```python
from build123d import *

# Parameters (mm, degrees)
SKETCH_1_R               = 19.5
SKETCH_1_R_2             = 18
EXTRUDE_1_DEPTH          = 20
SKETCH_3_R               = 27.5
EXTRUDE_2_DEPTH          = 3
SKETCH_10_R              = 6
SKETCH_10_R_2            = 5
EXTRUDE_6_DEPTH          = 10
CUT_EXTRUDE_4_DEPTH      = 19
CUT_EXTRUDE_4_DEPTH_BACK = 10
SKETCH_11_R              = 5.007506695
EXTRUDE_START            = 2
SKETCH_25_R              = 21.75
SKETCH_25_R_2            = 19.5
EXTRUDE_12_DEPTH         = 2
EXTRUDE_START_2          = -1
SKETCH_26_R              = 21.75
SKETCH_26_R_2            = 19.5
EXTRUDE_13_DEPTH         = 2
EXTRUDE_START_3          = -3
SKETCH_27_R              = 5.007506695
EXTRUDE_14_DEPTH         = 3
SKETCH_28_W              = 22.795630141
SKETCH_28_H              = 3
SKETCH_28_W_2            = 2.204369859
EXTRUDE_17_DEPTH         = 2
EXTRUDE_START_4          = -53
EXTRUDE_19_DEPTH         = 53
SKETCH_32_W              = 2.204369859
SKETCH_32_H              = 3
EXTRUDE_20_DEPTH         = 2
CUT_EXTRUDE_START        = -50
CUT_EXTRUDE_8_DEPTH      = 50


with BuildPart() as part:
    # Sketch 1 → Extrude 1 (new body)
    with BuildSketch(Plane(origin=(0, 0, 0), x_dir=(1, 0, 0), z_dir=(0, 1, 0))):
        with Locations(Location((0, 0, 0), (0, 0, 270))):
            Circle(SKETCH_1_R)
        with Locations(Location((0, 0, 0), (0, 0, 270))):
            Circle(SKETCH_1_R_2, mode=Mode.SUBTRACT)
    extrude(amount=EXTRUDE_1_DEPTH)

    # Sketch 3 → Extrude 2 (add)
    with BuildSketch(Plane.XZ):
        with Locations(Location((0, 0, 0), (0, 0, 270))):
            Circle(SKETCH_3_R)
    extrude(amount=EXTRUDE_2_DEPTH)

    # Sketch 10 → Extrude 6 (add)
    with BuildSketch(Plane(origin=(0, -3, 0), x_dir=(-1, 0, 0), z_dir=(0, -1, 0))):
        with Locations(Location((0, 11.196036894, 0), (0, 0, 90))):
            Circle(SKETCH_10_R)
        with Locations(Location((0, 11.196036894, 0), (0, 0, 90))):
            Circle(SKETCH_10_R_2, mode=Mode.SUBTRACT)
    extrude(amount=-EXTRUDE_6_DEPTH)

    # Sketch 11 → Cut-Extrude 4 (cut, two sides: drawn at the far end of the back side and taken through both)
    with BuildSketch(Plane(origin=(0, -3, 0), x_dir=(-1, 0, 0), z_dir=(0, -1, 0)).offset(-CUT_EXTRUDE_4_DEPTH_BACK)):
        with Locations(Location((0, 11.196036894, 0), (0, 0, 90))):
            Circle(SKETCH_11_R)
    extrude(amount=CUT_EXTRUDE_4_DEPTH + CUT_EXTRUDE_4_DEPTH_BACK, mode=Mode.SUBTRACT)

    # Sketch 25 → Extrude 12 (add)
    with BuildSketch(Plane(origin=(0, 7, 0), x_dir=(-1, 0, 0), z_dir=(0, -1, 0)).offset(EXTRUDE_START)):
        with Locations(Location((0, 0, 0), (0, 0, 90))):
            Circle(SKETCH_25_R)
        with Locations(Location((0, 0, 0), (0, 0, 90))):
            Circle(SKETCH_25_R_2, mode=Mode.SUBTRACT)
    extrude(amount=-EXTRUDE_12_DEPTH)

    # Sketch 26 → Extrude 13 (add)
    with BuildSketch(Plane(origin=(0, 10.5, 0), x_dir=(-1, 0, 0), z_dir=(0, -1, 0)).offset(EXTRUDE_START_2)):
        with Locations(Location((0, 0, 0), (0, 0, 90))):
            Circle(SKETCH_26_R)
        with Locations(Location((0, 0, 0), (0, 0, 90))):
            Circle(SKETCH_26_R_2, mode=Mode.SUBTRACT)
    extrude(amount=-EXTRUDE_13_DEPTH)

    # Sketch 27 → Extrude 14 (add)
    # profile 1 of 6: a face of its own
    with BuildSketch(Plane.XZ.offset(3).offset(EXTRUDE_START_3)):
        with BuildLine():
            Line((12.5, 0), (0, 0))
            Line((0, 0), (-12.5, 0))
            Line((-12.5, 0), (-12.5, -24.494897428))
            ThreePointArc((-12.5, -24.494897428), (-11.408888911, -25.021735628), (-10.295630141, -25.5))
            Line((-10.295630141, -25.5), (10.295630141, -25.5))
            ThreePointArc((10.295630141, -25.5), (11.408888911, -25.021735628), (12.5, -24.494897428))
            Line((12.5, -24.494897428), (12.5, 0))
        make_face()
        with Locations(Location((0, -11.196036894, 0), (0, 0, 270))):
            Circle(SKETCH_27_R, mode=Mode.SUBTRACT)
    # profile 2 of 6: a face of its own
    with BuildSketch(Plane.XZ.offset(3).offset(EXTRUDE_START_3)):
        with BuildLine():
            Line((-12.5, 0), (0, 0))
            Line((0, 0), (12.5, 0))
            Line((12.5, 0), (12.5, 24.494897428))
            ThreePointArc((12.5, 24.494897428), (11.408888911, 25.021735628), (10.295630141, 25.5))
            Line((10.295630141, 25.5), (-10.295630141, 25.5))
            ThreePointArc((-10.295630141, 25.5), (-11.408888911, 25.021735628), (-12.5, 24.494897428))
            Line((-12.5, 24.494897428), (-12.5, 0))
        make_face()
    # profile 3 of 6: a face of its own
    with BuildSketch(Plane.XZ.offset(3).offset(EXTRUDE_START_3)):
        with BuildLine():
            ThreePointArc((-10.295630141, -25.5), (-11.408888911, -25.021735628), (-12.5, -24.494897428))
            Line((-12.5, -24.494897428), (-12.5, -25.5))
            Line((-12.5, -25.5), (-10.295630141, -25.5))
        make_face()
    # profile 4 of 6: a face of its own
    with BuildSketch(Plane.XZ.offset(3).offset(EXTRUDE_START_3)):
        with BuildLine():
            Line((12.5, -25.5), (12.5, -24.494897428))
            ThreePointArc((12.5, -24.494897428), (11.408888911, -25.021735628), (10.295630141, -25.5))
            Line((10.295630141, -25.5), (12.5, -25.5))
        make_face()
    # profile 5 of 6: a face of its own
    with BuildSketch(Plane.XZ.offset(3).offset(EXTRUDE_START_3)):
        with BuildLine():
            ThreePointArc((10.295630141, 25.5), (11.408888911, 25.021735628), (12.5, 24.494897428))
            Line((12.5, 24.494897428), (12.5, 25.5))
            Line((12.5, 25.5), (10.295630141, 25.5))
        make_face()
    # profile 6 of 6: a face of its own
    with BuildSketch(Plane.XZ.offset(3).offset(EXTRUDE_START_3)):
        with BuildLine():
            Line((-12.5, 25.5), (-12.5, 24.494897428))
            ThreePointArc((-12.5, 24.494897428), (-11.408888911, 25.021735628), (-10.295630141, 25.5))
            Line((-10.295630141, 25.5), (-12.5, 25.5))
        make_face()
    extrude(amount=EXTRUDE_14_DEPTH)

    # Sketch 28 → Extrude 17 (add)
    with BuildSketch(Plane(origin=(0, 0, -25.5), x_dir=(-1, 0, 0), z_dir=(0, 0, -1))):
        with BuildLine():
            Line((12.5, -38), (12.5, -3))
            Line((12.5, -3), (10.295630141, -3))
            Line((10.295630141, -3), (-12.5, -3))
            Line((-12.5, -3), (-12.5, -38))
            Line((-12.5, -38), (-8.6, -38))
            Line((-8.6, -38), (-8.6, -37.5))
            ThreePointArc((-8.6, -37.5), (-7.1, -36), (-5.6, -37.5))
            Line((-5.6, -37.5), (-5.6, -38))
            Line((-5.6, -38), (-4, -38))
            ThreePointArc((-4, -38), (0, -34), (4, -38))
            Line((4, -38), (5.6, -38))
            Line((5.6, -38), (5.6, -37.5))
            ThreePointArc((5.6, -37.5), (7.1, -36), (8.6, -37.5))
            Line((8.6, -37.5), (8.6, -38))
            Line((8.6, -38), (12.5, -38))
        make_face()
        with Locations((-1.102184929, -1.5)):
            Rectangle(SKETCH_28_W, SKETCH_28_H)
        with Locations((11.397815071, -1.5)):
            Rectangle(SKETCH_28_W_2, SKETCH_28_H)
        with BuildLine():
            ThreePointArc((-12.5, -38), (0, -50.5), (12.5, -38))
            Line((12.5, -38), (8.6, -38))
            Line((8.6, -38), (8.6, -38.5))
            ThreePointArc((8.6, -38.5), (7.1, -40), (5.6, -38.5))
            Line((5.6, -38.5), (5.6, -38))
            Line((5.6, -38), (4, -38))
            ThreePointArc((4, -38), (0, -42), (-4, -38))
            Line((-4, -38), (-5.6, -38))
            Line((-5.6, -38), (-5.6, -38.5))
            ThreePointArc((-5.6, -38.5), (-7.1, -40), (-8.6, -38.5))
            Line((-8.6, -38.5), (-8.6, -38))
            Line((-8.6, -38), (-12.5, -38))
        make_face()
    extrude(amount=EXTRUDE_17_DEPTH)

    # Sketch 28_15 → Extrude 19 (add)
    with BuildSketch(Plane(origin=(0, 0, -25.5), x_dir=(-1, 0, 0), z_dir=(0, 0, -1)).offset(EXTRUDE_START_4)):
        with BuildLine():
            Line((12.5, -38), (12.5, -3))
            Line((12.5, -3), (10.295630141, -3))
            Line((10.295630141, -3), (-12.5, -3))
            Line((-12.5, -3), (-12.5, -38))
            Line((-12.5, -38), (-8.6, -38))
            Line((-8.6, -38), (-8.6, -37.5))
            ThreePointArc((-8.6, -37.5), (-7.1, -36), (-5.6, -37.5))
            Line((-5.6, -37.5), (-5.6, -38))
            Line((-5.6, -38), (-4, -38))
            ThreePointArc((-4, -38), (0, -34), (4, -38))
            Line((4, -38), (5.6, -38))
            Line((5.6, -38), (5.6, -37.5))
            ThreePointArc((5.6, -37.5), (7.1, -36), (8.6, -37.5))
            Line((8.6, -37.5), (8.6, -38))
            Line((8.6, -38), (12.5, -38))
        make_face()
        with BuildLine():
            ThreePointArc((-12.5, -38), (0, -50.5), (12.5, -38))
            Line((12.5, -38), (8.6, -38))
            Line((8.6, -38), (8.6, -38.5))
            ThreePointArc((8.6, -38.5), (7.1, -40), (5.6, -38.5))
            Line((5.6, -38.5), (5.6, -38))
            Line((5.6, -38), (4, -38))
            ThreePointArc((4, -38), (0, -42), (-4, -38))
            Line((-4, -38), (-5.6, -38))
            Line((-5.6, -38), (-5.6, -38.5))
            ThreePointArc((-5.6, -38.5), (-7.1, -40), (-8.6, -38.5))
            Line((-8.6, -38.5), (-8.6, -38))
            Line((-8.6, -38), (-12.5, -38))
        make_face()
    extrude(amount=EXTRUDE_19_DEPTH)

    # Sketch 32 → Extrude 20 (add)
    with BuildSketch(Plane.XY.offset(25.5)):
        with Locations((11.397815071, -1.5)):
            Rectangle(SKETCH_32_W, SKETCH_32_H)
        with Locations((-11.397815071, -1.5)):
            Rectangle(SKETCH_32_W, SKETCH_32_H)
    extrude(amount=EXTRUDE_20_DEPTH)

    # Sketch 28_18 → Cut-Extrude 8 (cut)
    with BuildSketch(Plane(origin=(0, 0, -25.5), x_dir=(-1, 0, 0), z_dir=(0, 0, -1)).offset(CUT_EXTRUDE_START)):
        with BuildLine():
            Line((12.5, -38), (12.5, -3))
            Line((12.5, -3), (10.295630141, -3))
            Line((10.295630141, -3), (-12.5, -3))
            Line((-12.5, -3), (-12.5, -38))
            Line((-12.5, -38), (-8.6, -38))
            Line((-8.6, -38), (-8.6, -37.5))
            ThreePointArc((-8.6, -37.5), (-7.1, -36), (-5.6, -37.5))
            Line((-5.6, -37.5), (-5.6, -38))
            Line((-5.6, -38), (-4, -38))
            ThreePointArc((-4, -38), (0, -34), (4, -38))
            Line((4, -38), (5.6, -38))
            Line((5.6, -38), (5.6, -37.5))
            ThreePointArc((5.6, -37.5), (7.1, -36), (8.6, -37.5))
            Line((8.6, -37.5), (8.6, -38))
            Line((8.6, -38), (12.5, -38))
        make_face()
        with BuildLine():
            ThreePointArc((-12.5, -38), (0, -50.5), (12.5, -38))
            Line((12.5, -38), (8.6, -38))
            Line((8.6, -38), (8.6, -38.5))
            ThreePointArc((8.6, -38.5), (7.1, -40), (5.6, -38.5))
            Line((5.6, -38.5), (5.6, -38))
            Line((5.6, -38), (4, -38))
            ThreePointArc((4, -38), (0, -42), (-4, -38))
            Line((-4, -38), (-5.6, -38))
            Line((-5.6, -38), (-5.6, -38.5))
            ThreePointArc((-5.6, -38.5), (-7.1, -40), (-8.6, -38.5))
            Line((-8.6, -38.5), (-8.6, -38))
            Line((-8.6, -38), (-12.5, -38))
        make_face()
    extrude(amount=CUT_EXTRUDE_8_DEPTH, mode=Mode.SUBTRACT)


solid = part.part
```
Source: CAD feature listing. Evaluate the final solid. Frame: model axes, mm. A direction names the side the tool comes from. Round coordinates to 2 decimals unless told otherwise and drop trailing zeros. Write each loop counter-clockwise with the first axis right and the second up, starting at its lowest first coordinate (ties: lowest second). Pieces come first, ordered by that corner, then holes. Notation, with made-up numbers: M -34,55 L -24,55 A34 ccw -24,93 Z; hole C 69,51 d7. An arc over 180 degrees is marked long. Answer as a JSON object with one key per item and string values. Group by question number.
(1) Mould query, pull axis Z, two halves, no side actions, for faces 1 (the cylindrical face through (0.275, -50.497, 26.021)), 2 (the flat face through (0, 0, 0)), 3 (the cylindrical face through (19.334, 2.465, -2.539)). Classes: +Z half, -Z half, draft (parallel to the pull), parting line (faces both ways), or undercut.
(2) Section query D-D on x = 15. Output: boundary loops of the cut face in (y, z).
(3) First-contact query: pin 1 (5 mm diameter, centred on x = -8.5, z = 5.5, fed in from -Y); pin 2 (0.5 mm diameter, centred on y = -38, z = -27, fed in from -X); pin 3 (2 mm diameter, centred on x = -5, z = 26.5, fed in from +Y); pin 4 (10.5 mm diameter, centred on x = 0, y = -38, fed in from -Z). Flat tips, straight axial feed; report the tip coordinate or a pass-through.
(4) Section query B-B on z = 10. Output: boundary loops of the cut face in (x, y).
(5) Section query A-A on y = -6. Output: boundary loops of the cut face in (x, z), then the cut area to 3 significant figures.
(6) Reachability of faces 4 (the flat face through (-5, 7, -13)), 5 (the cylindrical face through (7.1, -40, -26.5)), 6 (the flat face through (18, 5, 8)) from +Z, -Z, +X, -X, +Y, -Y: full face, straight path, thin tool, end or side. Return the list, or none.
(7) Ray query, line 1 (X direction, y = -38, z = 25.4); line 2 (Y direction, x = 0, z = 25); line 3 (X direction, y = 9, z = 0). Return the intervals inside material, ascending. Write a range as [from, to].
(8) Section query C-C on y = -35. Output: boundary loops of the cut face in (x, z).
Computed values:
{
 "1": {"face 1": "draft", "face 2": "undercut", "face 3": "parting line"},
 "2": {"outline": "M -3,-23.05 L 0,-23.05 L 0,-12.46 L 5,-12.46 L 5,-15.75 L 7,-15.75 L 7,-12.46 L 11.5,-12.46 L 11.5,-15.75 L 13.5,-15.75 L 13.5,-12.46 L 20,-12.46 L 20,-9.95 L 0,-9.95 L 0,9.95 L 20,9.95 L 20,12.46 L 13.5,12.46 L 13.5,15.75 L 11.5,15.75 L 11.5,12.46 L 7,12.46 L 7,15.75 L 5,15.75 L 5,12.46 L 0,12.46 L 0,23.05 L -3,23.05 Z"},
 "3": {"pin 1": "y = -3", "pin 2": "x = -12.5", "pin 3": "y = 0", "pin 4": "z = -27.5"},
 "4": {"outline": "M -25.62,-3 L 25.62,-3 L 25.62,0 L 16.74,0 L 16.74,5 L 19.31,5 L 19.31,7 L 16.74,7 L 16.74,11.5 L 19.31,11.5 L 19.31,13.5 L 16.74,13.5 L 16.74,20 L 14.97,20 L 14.97,0 L -14.97,0 L -14.97,20 L -16.74,20 L -16.74,13.5 L -19.31,13.5 L -19.31,11.5 L -16.74,11.5 L -16.74,7 L -19.31,7 L -19.31,5 L -16.74,5 L -16.74,0 L -25.62,0 Z"},
 "5": {"outline": "M -12.5,-27.5 L 12.5,-27.5 L 12.5,-25.5 L -12.5,-25.5 Z; M -12.5,24.5 L 12.5,24.5 L 12.5,27.5 L -12.5,27.5 Z", "area": "125 mm^2"},
 "6": {"face 4": "+Y", "face 5": "+Z, -Z", "face 6": "none"},
 "7": {"line 1": "[-12.5, -8.6], [-5.6, -4], [4, 5.6], [8.6, 12.5]", "line 2": "[-50.5, -42], [-34, 0]", "line 3": "[-19.5, -18], [18, 19.5]"},
 "8": {"outline": "M -12.5,-27.5 L -2.65,-27.5 L -2.65,-25.5 L -12.5,-25.5 Z; M -12.5,24.5 L -2.65,24.5 L -2.65,27.5 L -12.5,27.5 Z; M 2.65,-27.5 L 12.5,-27.5 L 12.5,-25.5 L 2.65,-25.5 Z; M 2.65,24.5 L 12.5,24.5 L 12.5,27.5 L 2.65,27.5 Z"}
}
